Read the model definition and answer for the solid it produces. Units are mm, in the model's axes. A direction names the side the tool comes from. Coordinates: 2 decimals unless noted, no trailing zeros. Order: outer loops, then holes, each group sorted by start corner. A loop starts at its lowest first (then second) coordinate and runs counter-clockwise, first axis right, second up. Notation, with made-up numbers: (-9, 51.5) -> (34, 51.5) arc R18 cw to (34, 75.5) -> close; hole circle Ø6 at (20, 55.5). An arc over 180 degrees is marked (long way). Answer in a Markdown table with one row per item.
from build123d import *

# Parameters (mm, degrees)
SKETCH1_W           = 86.120484183
SKETCH1_H           = 54.608623026
SKETCH1_W_2         = 2.7
SKETCH1_H_2         = 2.7
SKETCH1_W_3         = 6
SKETCH1_H_3         = 2.65
BOSS_EXTRUDE1_DEPTH = 3


with BuildPart() as part:
    # Sketch1 → Boss-Extrude1 (new body)
    with BuildSketch(Plane(origin=(0, 0, 0), x_dir=(1, 0, 0), z_dir=(0, 1, 0))):
        with Locations((155.479789649, -59.671038124)):
            Rectangle(SKETCH1_W, SKETCH1_H)
        with Locations((193.834702188, -55.435925566)):
            Rectangle(SKETCH1_W_2, SKETCH1_H_2, mode=Mode.SUBTRACT)
        with Locations((193.933836211, -49.435925566)):
            Rectangle(SKETCH1_W_2, SKETCH1_H_2, mode=Mode.SUBTRACT)
        with Locations((193.933836211, -43.435925566)):
            Rectangle(SKETCH1_W_2, SKETCH1_H_2, mode=Mode.SUBTRACT)
        with Locations((187.484702188, -54.885926943)):
            Rectangle(SKETCH1_W_3, SKETCH1_H_3, mode=Mode.SUBTRACT)
        with Locations((187.583836211, -43.985925566)):
            Rectangle(SKETCH1_W_3, SKETCH1_H_3, mode=Mode.SUBTRACT)
        Polygon((129.433836211, -75.435925566), (132.733836211, -75.435925566), (132.733836211, -72.735925566), (135.433836211, -72.735925566), (135.433836211, -75.435925566), (138.733836211, -75.435925566), (138.733836211, -72.735925566), (141.433836211, -72.735925566), (141.433836211, -75.435925566), (146.733836211, -75.435925566), (146.733836211, -72.735925566), (149.433836211, -72.735925566), (149.433836211, -75.435925566), (152.733836211, -75.435925566), (152.733836211, -72.735925566), (155.433836211, -72.735925566), (155.433836211, -75.435925566), (158.733836211, -75.435925566), (158.733836211, -72.735925566), (161.433836211, -72.735925566), (161.433836211, -75.435925566), (165.083836211, -75.435925566), (165.083836211, -73.785925566), (162.383836211, -73.785925566), (162.383836211, -71.085925566), (165.083836211, -71.085925566), (165.083836211, -67.785925566), (162.383836211, -67.785925566), (162.383836211, -65.085925566), (165.083836211, -65.085925566), (165.083836211, -61.785925566), (162.383836211, -61.785925566), (162.383836211, -59.085925566), (165.083836211, -59.085925566), (165.083836211, -37.002032915), (170.083836211, -37.002032915), (170.083836211, -59.085925566), (172.783836211, -59.085925566), (172.783836211, -61.785925566), (170.083836211, -61.785925566), (170.083836211, -65.085925566), (172.783836211, -65.085925566), (172.783836211, -67.785925566), (170.083836211, -67.785925566), (170.083836211, -71.085925566), (172.783836211, -71.085925566), (172.783836211, -73.785925566), (170.083836211, -73.785925566), (170.083836211, -75.435925566), (170.083836211, -80.435925566), (161.433836211, -80.435925566), (161.433836211, -83.135925566), (158.733836211, -83.135925566), (158.733836211, -80.435925566), (155.433836211, -80.435925566), (155.433836211, -83.135925566), (152.733836211, -83.135925566), (152.733836211, -80.435925566), (149.433836211, -80.435925566), (149.433836211, -83.135925566), (146.733836211, -83.135925566), (146.733836211, -80.435925566), (141.433836211, -80.435925566), (141.433836211, -83.135925566), (138.733836211, -83.135925566), (138.733836211, -80.435925566), (135.433836211, -80.435925566), (135.433836211, -83.135925566), (132.733836211, -83.135925566), (132.733836211, -80.435925566), (129.433836211, -80.435925566), (129.433836211, -83.135925566), (126.733836211, -83.135925566), (126.733836211, -80.435925566), (116.63506554, -80.435925566), (116.63506554, -75.435925566), (126.733836211, -75.435925566), (126.733836211, -72.735925566), (129.433836211, -72.735925566), align=None, mode=Mode.SUBTRACT)
    extrude(amount=BOSS_EXTRUDE1_DEPTH)


solid = part.part
Q1. For a pull along X with two mould halves and no side action, classify faces 3 (the face through (163, 1, 75.436)), 4 (the face through (134, 1, 72.736)), 5 (the face through (112.42, 1, 60)), 6 (the face through (198.54, 1, 60)) as pulls with the +X half, pulls with the -X half, needs draft (parallel to the pull), parting line crosses it, or undercut.
Outcome:
| item | result |
|---|---|
| face 3 | undercut |
| face 4 | undercut |
| face 5 | pulls with the -X half |
| face 6 | pulls with the +X half |
Q2. The part is cut by section D-D (y = 2.15). Give the number of separate pieces and of enclosed holes in the cut face, then the cut area to 3 significant figures.
Outcome:
| item | result |
|---|---|
| separate pieces | 1 |
| enclosed holes | 6 |
| area | 4,060 mm² |
Q3. The part is cut by section B-B (z = 60). Write down the section's boundary in (x, y), then the cut area to 3 significant figures.
Outcome:
| item | result |
|---|---|
| outline | (112.42, 0) -> (162.38, 0) -> (162.38, 3) -> (112.42, 3) -> close; (172.78, 0) -> (198.54, 0) -> (198.54, 3) -> (172.78, 3) -> close |
| area | 227 mm² |
Q4. The part is cut by section C-C (x = 137.5). Write down the section's boundary in (y, z), then the cut area to 3 significant figures.
Outcome:
| item | result |
|---|---|
| outline | (0, 32.37) -> (3, 32.37) -> (3, 75.44) -> (0, 75.44) -> close; (0, 80.44) -> (3, 80.44) -> (3, 86.98) -> (0, 86.98) -> close |
| area | 149 mm² |
Q5. Consider line 1 (Z direction, x = 162.5, y = 0.85); line 2 (X direction, y = 0.5, z = 54.5); line 3 (Z direction, x = 190, y = 2.75). Determine where each line is inside the solid, lowest interval first.
Outcome:
| item | result |
|---|---|
| line 1 | 32.37 to 59.09, 61.79 to 65.09, 67.79 to 71.09, 73.79 to 75.44, 80.44 to 86.98 |
| line 2 | 112.42 to 165.08, 170.08 to 184.48, 190.48 to 192.48, 195.18 to 198.54 |
| line 3 | 32.37 to 42.66, 45.31 to 53.56, 56.21 to 86.98 |
Q6. For faces 1 (the face through (155, 3, 59)), 2 (the face through (157, 1, 75.436)), determine the directions among +Z, -Z, +X, -X, +Y, -Y from which every point of the face is accessible in a straight line to the end or side of a thin tool.
Outcome:
| item | result |
|---|---|
| face 1 | +Z, -Z, +X, -X, +Y |
| face 2 | +Y, -Y |
Q7. The part is cut by section A-A (x = 186). Write down the section's boundary in (y, z), then the cut area to 3 significant figures.
Outcome:
| item | result |
|---|---|
| outline | (0, 32.37) -> (3, 32.37) -> (3, 42.66) -> (0, 42.66) -> close; (0, 45.31) -> (3, 45.31) -> (3, 53.56) -> (0, 53.56) -> close; (0, 56.21) -> (3, 56.21) -> (3, 86.98) -> (0, 86.98) -> close |
| area | 148 mm² |
